from build123d import *

# Parameters (mm, degrees)
ESBO_O1_W                = 72
ESBO_O1_H                = 35
RESSALTO_EXTRUS_O1_DEPTH = 23
CORTE_EXTRUS_O1_DEPTH    = 0.5
FILETE1_R                = 2


with BuildPart() as part:
    # Esboço1 → Ressalto-extrusão1 (new body)
    with BuildSketch(Plane.XY):
        Rectangle(ESBO_O1_W, ESBO_O1_H)
    extrude(amount=RESSALTO_EXTRUS_O1_DEPTH)

    # Esboço2 → Corte-extrusão1 (cut)
    with BuildSketch(Plane(origin=(36, 0, 0), x_dir=(0, 0, -1), z_dir=(1, 0, 0))):
        with BuildLine():
            Line((-4, 6), (-4, -6))
            ThreePointArc((-4, -6), (-11.5, -13.5), (-19, -6))
            Line((-19, -6), (-19, 6))
            ThreePointArc((-19, 6), (-11.5, 13.5), (-4, 6))
        make_face()
    corte_extrus_o1 = extrude(amount=-CORTE_EXTRUS_O1_DEPTH, mode=Mode.SUBTRACT)

    # Espelhar1: Corte-extrusão1 across plane
    add(corte_extrus_o1.mirror(Plane(origin=(0, 0, 0), x_dir=(0, 0, 1), z_dir=(1, 0, 0))), mode=Mode.SUBTRACT)

    # Filete1
    filete1_edges = [part.edges().sort_by_distance(p)[0] for p in [
        (-36, 0, 23),
        (0, -17.5, 23),
        (36, 0, 23),
        (0, -17.5, 0),
        (-36, 0, 0),
        (0, 17.5, 0),
        (36, 0, 0),
        (0, 17.5, 23),
        (36, -17.5, 11.5),
        (-36, -17.5, 11.5),
        (-36, 17.5, 11.5),
        (36, 17.5, 11.5),
    ]]
    fillet(filete1_edges, radius=FILETE1_R)


solid = part.part
Can you work these out from the model? Positions are in its coordinate system, mm. A direction names the side the tool comes from. Give positions to 0.01 mm unless a question says otherwise; leave off trailing zeros. Answer as a JSON object with one key per item and string values.
Q1. If we mould it in two halves opening along Y, with no side actions, what happens to faces 4 (the cylindrical face through (-35.75, 13.5, 11.66)), 5 (the cylindrical face through (-35.43, -16.9, 11.63)), 6 (the flat face through (0, 17.5, 11))? For each: pulls with the +Y half, pulls with the -Y half, needs draft (parallel to the pull), parting line crosses it, or undercut.
Geometry says:
{"face 4": "undercut", "face 5": "pulls with the -Y half", "face 6": "pulls with the +Y half"}
Q2. If I drill on L1, parallel to X at y = -10, z = 16.5; L2, parallel to X at y = -14.5, z = 1, over which ranges is the centre line in solid material (lowest first)?
Geometry says:
{"L1": "-35.5 to 35.5", "L2": "-35.73 to 35.73"}
Q3. Which directions (+Z, -Z, +X, -X, +Y, -Y) give clear straight access to the entire face, cutting with the end or side of a thin tool? Please do faces 1 (the cylindrical face through (-35.43, 0.22, 22.4)), 2 (the flat face through (35.5, 0, 11)), 3 (the flat face through (-35.5, 0, 11)).
Geometry says:
{"face 1": "+Z, -X, +Y, -Y", "face 2": "+X", "face 3": "-X"}
Q4. Will these pins go through, and if not, where does the flat tip stop? P1, Ø12, axis at y = 6, z = 12.5, coming from the +X side; P2, Ø7.5, axis at y = -3.5, z = 11.5, coming from the -X side; P3, Ø0.6, axis at x = 36, y = 0.5, coming from the +Z side.
Geometry says:
{"P1": "x = 35.5", "P2": "x = -35.5", "P3": "z = 22.05"}
